Here's how the part is built. I have some questions about the finished solid (model axes, mm). Coordinates: 2 decimals unless noted, no trailing zeros. Order: outer loops, then holes, each group sorted by start corner. A loop starts at its lowest first (then second) coordinate and runs counter-clockwise, first axis right, second up. Notation, with made-up numbers: (70.25, -37) -> (83.25, -37) arc R22 ccw to (83.25, -12) -> close; hole circle Ø4 at (-2.5, 18.25). An arc over 180 degrees is marked (long way). One line per item, written item: value. Start each with the question number.
```python
from build123d import *

# Parameters (mm, degrees)
F1_DEPTH = 4
F2_R     = 3.99999


# Not quite as in the source:
# - a fillet or chamfer is up to 0.001 mm smaller than in the source, because OpenCascade refuses the exact size


with BuildPart() as f1:
    # F0 (on Top) → F1 (new body)
    with BuildSketch(Plane.XY):
        with BuildLine():
            Line((6.2132034356, -15), (163.3772233983, -15))
            ThreePointArc((163.3772233983, -15), (230, 0), (163.3772233983, 15))
            Line((163.3772233983, 15), (6.2132034356, 15))
            Line((6.2132034356, 15), (-104.9185408386, 126.1317442742))
            ThreePointArc((-104.9185408386, 126.1317442742), (-162.6345596729, 162.6345596729), (-126.1317442742, 104.9185408386))
            Line((-126.1317442742, 104.9185408386), (-21.2132034356, 0))
            Line((-21.2132034356, 0), (-126.1317442742, -104.9185408386))
            ThreePointArc((-126.1317442742, -104.9185408386), (-162.6345596729, -162.6345596729), (-104.9185408386, -126.1317442742))
            Line((-104.9185408386, -126.1317442742), (6.2132034356, -15))
        make_face()
    extrude(amount=F1_DEPTH)

    # F2 (radius 4 in the source; OpenCascade refuses exactly that, so slightly less here)
    f2_edges = [f1.edges().sort_by_distance(p)[0] for p in [
        (-49.352669, -70.565872, 4),
        (84.795213, -15, 4),
        (230, 0, 4),
        (84.795213, 15, 4),
        (-49.352669, 70.565872, 4),
        (-162.63456, 162.63456, 4),
        (-73.672474, 52.45927, 4),
        (-73.672474, -52.45927, 4),
        (-162.63456, -162.63456, 4),
    ]]
    fillet(f2_edges, radius=F2_R)


solid = f1.part
```
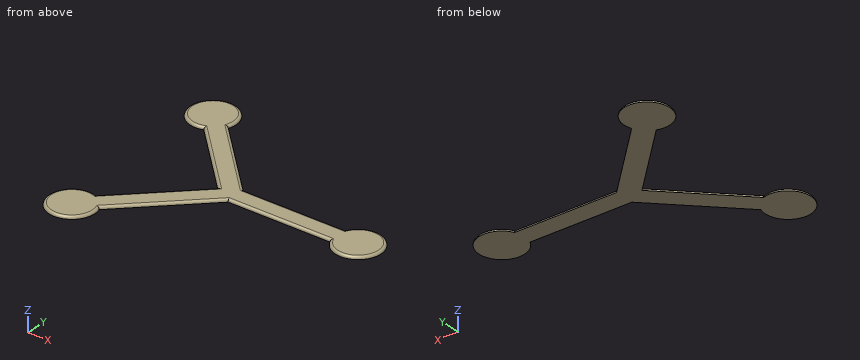
Q1. I need wall thicknesses on line 1 (Y direction, x = 26, z = 0.4); line 2 (Y direction, x = -100, z = 0.2); line 3 (X direction, y = 32, z = 0.7). Which ranges of each line are inside material? Lowest first, please.
Q2. For P1, Ø1.5, axis at x = -102, z = 0.5, coming from the -Y side, with a flat end and sliding along its axis, tell me the tip position at first contact or that it passes through.
Q3. Imagine slicing it at B-B (z = 2.45). Write out the boundary of the cut face in (x, y), plus the area to 3 significant figures.
Completed:
1. line 1: y = -14.98 to 14.98
1. line 2: y = -121.21 to -78.79, 78.79 to 121.21
1. line 3: x = -53.13 to -10.87, 180.98 to 209.02
2. P1: stops at y = -123.93
3. outline: (-125.92, -105.89) arc R34.16 ccw (long way) to (-105.89, -125.92) -> (5.87, -14.16) -> (163.91, -14.16) arc R34.16 ccw (long way) to (163.91, 14.16) -> (5.87, 14.16) -> (-105.89, 125.92) arc R34.16 ccw (long way) to (-125.92, 105.89) -> (-20.03, 0) -> close
3. area: 24,400 mm2
